```python
from build123d import *

# Parameters (mm, degrees)
BOSS_EXTRUDE1_DEPTH        = 3
SKETCH2_W                  = 9.75
SKETCH2_H                  = 10
BOSS_EXTRUDE2_DEPTH        = 6.75
SKETCH3_W                  = 6.75
SKETCH3_H                  = 3.5
CUT_EXTRUDE1_DEPTH         = 5
SKETCH4_W                  = 4.75
SKETCH4_H                  = 10
BOSS_EXTRUDE3_DEPTH        = 35.25
SKETCH5_W                  = 4.75
SKETCH5_H                  = 6.5
BOSS_EXTRUDE4_DEPTH        = 5
F_2_0_2_DIAMETER_HOLE1_D   = 2
F_3_2_3_2_DIAMETER_HOLE1_D = 3.2
FILLET1_R                  = 1
FILLET2_R                  = 2.25
FILLET3_R                  = 3


with BuildPart() as part:
    # Sketch1 → Boss-Extrude1 (new body)
    with BuildSketch(Plane(origin=(-25, 0, 0), x_dir=(0, -1, 0), z_dir=(-1, 0, 0))):
        with BuildLine():
            Line((-6.5, -2.25), (0, -2.25))
            Line((0, -2.25), (5.014501105, -4.64943299))
            ThreePointArc((5.014501105, -4.64943299), (10.980645857, -2.805310946), (9.610876171, 3.287258325))
            Line((9.610876171, 3.287258325), (3.5, 7.5))
            Line((3.5, 7.5), (-6.5, 7.5))
            Line((-6.5, 7.5), (-6.5, -2.25))
        make_face()
    extrude(amount=-BOSS_EXTRUDE1_DEPTH)

    # Sketch2 → Boss-Extrude2 (add)
    with BuildSketch(Plane(origin=(-22, 0, 0), x_dir=(0, 0, -1), z_dir=(1, 0, 0))):
        with Locations((-2.625, 1.5)):
            Rectangle(SKETCH2_W, SKETCH2_H)
    extrude(amount=BOSS_EXTRUDE2_DEPTH)

    # Sketch3 → Cut-Extrude1 (cut)
    with BuildSketch(Plane(origin=(0, 0, -2.25), x_dir=(-1, 0, 0), z_dir=(0, 0, -1))):
        with Locations((18.625, -1.75)):
            Rectangle(SKETCH3_W, SKETCH3_H)
    extrude(amount=-CUT_EXTRUDE1_DEPTH, mode=Mode.SUBTRACT)

    # Sketch4 → Boss-Extrude3 (add)
    with BuildSketch(Plane(origin=(-15.25, 0, 0), x_dir=(0, 0, -1), z_dir=(1, 0, 0))):
        with Locations((-5.125, 1.5)):
            Rectangle(SKETCH4_W, SKETCH4_H)
    extrude(amount=BOSS_EXTRUDE3_DEPTH)

    # Sketch5 → Boss-Extrude4 (add)
    with BuildSketch(Plane(origin=(0, 0, 2.75), x_dir=(-1, 0, 0), z_dir=(0, 0, -1))):
        with Locations((-17.625, 3.25)):
            Rectangle(SKETCH5_W, SKETCH5_H)
    extrude(amount=BOSS_EXTRUDE4_DEPTH)

    # Ø2.0 (2) Diameter Hole1 (through all)
    with Locations(Plane(origin=(0, 0, 0), x_dir=(-1, 0, 0), z_dir=(0, -1, 0))):
        with Locations((-17.5, 0), (17.5, 0)):
            Hole(F_2_0_2_DIAMETER_HOLE1_D / 2)

    # Ø3.2 (3.2) Diameter Hole1 (through all)
    with Locations(Plane(origin=(-22, 0, 0), x_dir=(0, 0, -1), z_dir=(1, 0, 0))):
        with Locations((0.5, -7)):
            Hole(F_3_2_3_2_DIAMETER_HOLE1_D / 2)

    # Fillet1
    fillet1_edges = [part.edges().sort_by_distance(p)[0] for p in [
        (20, -1.75, 2.75),
        (20, 3.25, -2.25),
    ]]
    fillet(fillet1_edges, radius=FILLET1_R)

    # Fillet2
    fillet2_edges = [part.edges().sort_by_distance(p)[0] for p in [
        (-15.25, 3.25, -2.25),
        (15.25, 3.25, -2.25),
    ]]
    fillet(fillet2_edges, radius=FILLET2_R)

    # Fillet3
    fillet3_edges = [part.edges().sort_by_distance(p)[0] for p in [
        (20, 1.5, 7.5),
        (-25, 3.25, -2.25),
        (-25, 1.5, 7.5),
    ]]
    fillet(fillet3_edges, radius=FILLET3_R)


solid = part.part
```
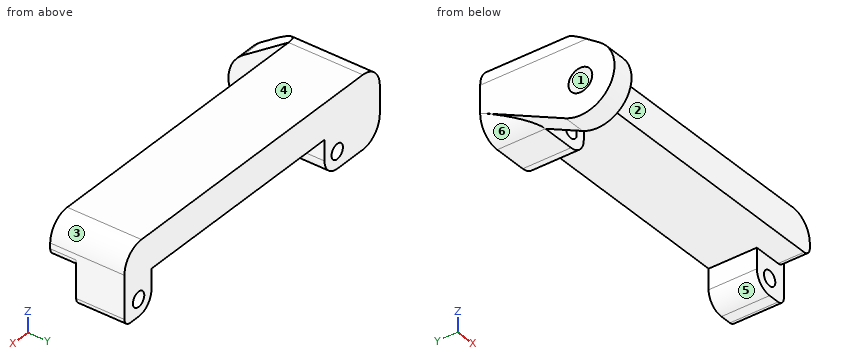
Geometry check sheet. Reference: the model listing, model coordinates, mm. Face numbers are marked on the shaded views. A direction names the side the tool comes from. Coordinates: 2 decimals unless noted, no trailing zeros. Order: outer loops, then holes, each group sorted by start corner. A loop starts at its lowest first (then second) coordinate and runs counter-clockwise, first axis right, second up. Notation, with made-up numbers: M 77,19.5 L 96,19.5 A7 cw 96,25.5 Z; hole C 5,26 d6. An arc over 180 degrees is marked long. One line per question, with ' | ' between items. Start each with the question number.
Item 1: Set-up check for the marked faces 4, 5 and 6: record each of +Z, -Z, +X, -X, +Y, -Y from which the full face is reachable in a straight line by a thin tool's end or side.
Item 2: Material ranges on L1, parallel to Y at x = -24, z = -0.5; L2, parallel to Z at x = -17.5, y = 2.5; L3, parallel to X at y = 4, z = -0.25, recorded low to high. Write a range as [from, to].
Item 3: Cross-section at D-D on y = 2.5. Enter the section's corners in (x, z), then the cut area to 3 significant figures.
Item 4: Draft check along Y on the marked faces 1, 2 and 3. Enter one of: pulls with the +Y half, pulls with the -Y half, needs draft (parallel to the pull), parting line crosses it, or undercut.
Item 5: Gauge pin test, flat ends, axial feed: pin 1 (4 mm diameter, centred on x = 18.5, z = -0.5, fed in from -Y); pin 2 (3 mm diameter, centred on x = 17.5, z = 0, fed in from +Y); pin 3 (1.3 mm diameter, centred on x = -21, y = 5, fed in from -Z); pin 4 (5 mm diameter, centred on y = -7, z = -0.5, fed in from +X). Record the tip position at first contact, or that the pin passes through.
Item 6: Cross-section at B-B on y = -6.25. Enter the section's corners in (x, z), then the cut area to 3 significant figures.
Item 7: Cross-section at C-C on z = -0.5. Enter the section's corners in (x, y), then the cut area to 3 significant figures.
Item 8: Cross-section at A-A on z = 2.25. Enter the section's corners in (x, y), then the cut area to 3 significant figures.
Findings:
1) face 4: +Z, +X, -X, +Y, -Y | face 5: -Z, +Y, -Y | face 6: -Z, -X, +Y
2) L1: y = [-11.6, -8.6], [-5.4, 6.5] | L2: z = [-2.25, -1], [1, 7.5] | L3: x = [-25, -18.47], [-16.53, -15.26], [15.26, 16.53], [18.47, 20]
3) outline: M -25,-1.05 L -24.4,-1.05 A3 ccw -22,-2.25 L -17.5,-2.25 A2.25 ccw -15.25,0 L -15.25,2.75 L 15.25,2.75 L 15.25,0 A2.25 ccw 17.5,-2.25 L 19,-2.25 A1 ccw 20,-1.25 L 20,4.5 A3 ccw 17,7.5 L -22,7.5 A3 ccw -25,4.5 Z; hole C -17.5,0 d2; hole C 17.5,0 d2 | area: 272 mm²
4) face 1: undercut | face 2: pulls with the -Y half | face 3: needs draft
5) pin 1: stops at y = 0 | pin 2: stops at y = 6.5 | pin 3: stops at z = -2.25 | pin 4: stops at x = -22
6) outline: M -25,-5.04 L -22,-5.04 L -22,-1.91 L -25,-1.91 Z; M -25,0.91 L -22,0.91 L -22,5.6 L -24.79,5.6 A3 ccw -25,4.5 Z | area: 23.4 mm²
7) outline: M -25,-11.6 L -22,-11.6 L -22,-8.6 L -25,-8.6 Z; M -25,-5.4 L -22,-5.4 L -22,0 L -18.37,0 L -18.37,6.5 L -24.73,6.5 L -24.73,3.66 L -25,3.66 Z; M -16.63,0 L -15.31,0 L -15.31,6.5 L -16.63,6.5 Z; M 15.31,0 L 16.63,0 L 16.63,6.5 L 15.31,6.5 Z; M 18.37,0 L 20,0 L 20,6.5 L 18.37,6.5 Z | area: 95.4 mm²
8) outline: M -25,-10.69 L -22,-10.69 L -22,0 L -15.25,0 L -15.25,6.5 L -25,6.5 Z; M 15.25,0 L 20,0 L 20,6.5 L 15.25,6.5 Z | area: 126 mm²
